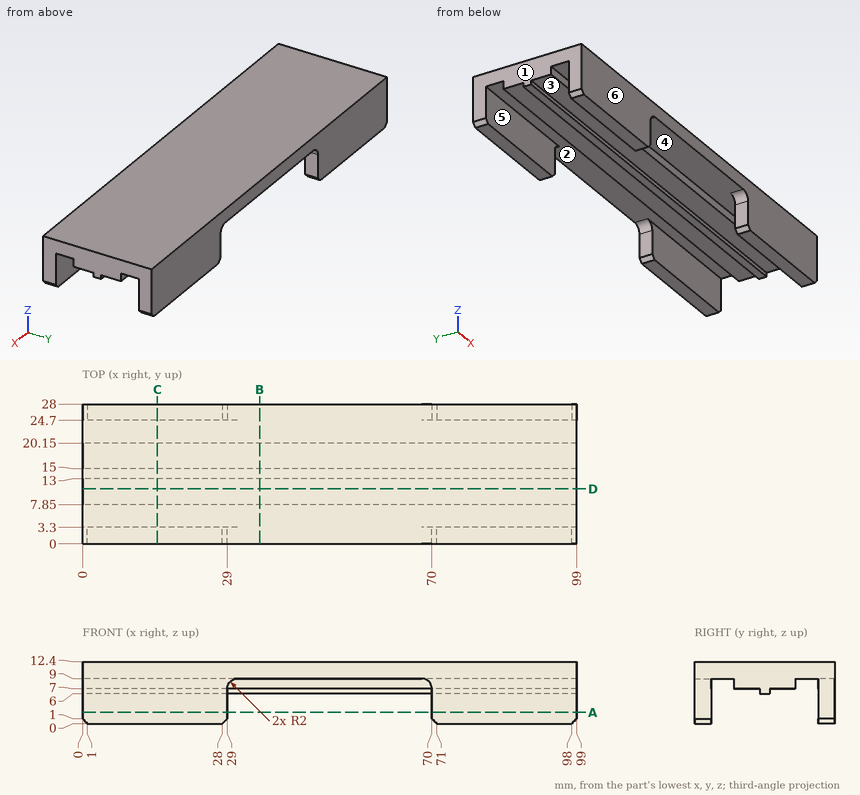
Can you work these out from the drawing? Everything is in mm from the part's minimum corner. A direction names the side the tool comes from. Coordinates: 2 decimals unless noted, no trailing zeros. Order: outer loops, then holes, each group sorted by start corner. A loop starts at its lowest first (then second) coordinate and runs counter-clockwise, first axis right, second up. Notation, with made-up numbers: (-39.5, 64) -> (-24.5, 64) arc R25 cw to (-24.5, 84) -> close; hole circle Ø2 at (-4, 5.5). An arc over 180 degrees is marked (long way). Return JSON: item names as keys, results as strings.
1) On a 3-axis mill with a long thin cutter (end or side, diameter ignored), from which of +Z, -Z, +X, -X, +Y, -Y can I reach the whole of each face in a straight line? I mean the marked faces 5 and 6. Say none if no direction works.
Conclusion:
{"face 5": "-Z, +X, -X", "face 6": "+Z, -Z, +X, -X, -Y"}
2) If I drill on probe 1 along Y at (x, z) = (91, 8.25); probe 2 along Y at (x, z) = (92.5, 6.75); probe 3 along Y at (x, z) = (83, 4.25), over which ranges is the centre line in solid material (lowest first)?
Conclusion:
{"probe 1": "y = 0 to 3.3, 7.85 to 20.15, 24.7 to 28", "probe 2": "y = 0 to 3.3, 13 to 15, 24.7 to 28", "probe 3": "y = 0 to 3.3, 24.7 to 28"}
3) If we section it at A-A on z = 2.25: List the corners of the cut face in (x, y) for me, plus the area to 3 significant figures.
Conclusion:
{"outline": "(0, 0) -> (29, 0) -> (29, 3.3) -> (0, 3.3) -> close; (0, 24.7) -> (29, 24.7) -> (29, 28) -> (0, 28) -> close; (70, 0) -> (99, 0) -> (99, 3.3) -> (70, 3.3) -> close; (70, 24.7) -> (99, 24.7) -> (99, 28) -> (70, 28) -> close", "area": "383 mm²"}
4) If we section it at D-D on y = 11: List the corners of the cut face in (x, z) for me, plus the area to 3 significant figures.
Conclusion:
{"outline": "(0, 7) -> (99, 7) -> (99, 12.4) -> (0, 12.4) -> close", "area": "535 mm²"}
5) If we section it at B-B on x = 35.5: List the corners of the cut face in (y, z) for me.
Conclusion:
{"outline": "(0, 9) -> (7.85, 9) -> (7.85, 7) -> (13, 7) -> (13, 6) -> (15, 6) -> (15, 7) -> (20.15, 7) -> (20.15, 9) -> (28, 9) -> (28, 12.4) -> (0, 12.4) -> close"}
6) If we section it at C-C on x = 15: List the corners of the cut face in (y, z) for me.
Conclusion:
{"outline": "(0, 0) -> (3.3, 0) -> (3.3, 9) -> (7.85, 9) -> (7.85, 7) -> (13, 7) -> (13, 6) -> (15, 6) -> (15, 7) -> (20.15, 7) -> (20.15, 9) -> (24.7, 9) -> (24.7, 0) -> (28, 0) -> (28, 12.4) -> (0, 12.4) -> close"}
7) I'm going to push flat-ended pins straight in: P1, Ø5.5, axis at x = 52, y = 17, coming from the -Z side; P2, Ø6, axis at x = 25, z = 5.5, coming from the -Y side; P3, Ø1.1, axis at x = 68, z = 6.5, coming from the +Y side; P4, Ø2.5, axis at x = 48, y = 23, coming from the -Z side. Where does each tip first touch, or does it pass through?
Conclusion:
{"P1": "stops at z = 6", "P2": "stops at y = 0", "P3": "stops at y = 20.15", "P4": "stops at z = 9"}
8) Thinking about a two-plate mould opening in X: for the marked faces 1, 2, 3 and 4, which applies, +X half, -X half, draft (parallel to the pull), parting line (faces both ways), or undercut?
Conclusion:
{"face 1": "-X half", "face 2": "undercut", "face 3": "draft", "face 4": "undercut"}
